```python
from build123d import *

# Parameters (mm, degrees)
F0_W     = 117.5
F0_H     = 117.5
F1_DEPTH = 150
F2_R     = 8.3617608376
F3_DEPTH = 50.8
F4_T     = -2.54


with BuildPart() as f1:
    # F0 (on Top) → F1 (new body)
    with BuildSketch(Plane.XY):
        with Locations((2.2854433954, -9.9431091547)):
            Rectangle(F0_W, F0_H)
    extrude(amount=F1_DEPTH)

    # F2 (on face) → F3 (join)
    with BuildSketch(Plane.XY.offset(150)):
        with Locations((0, 10.8060371131)):
            Circle(F2_R)
    extrude(amount=F3_DEPTH)

    # F4
    f4_openings = [f1.faces().sort_by_distance(p)[0] for p in [
        (0, 10.806037, 200.8),
    ]]
    offset(amount=F4_T, openings=f4_openings, kind=Kind.INTERSECTION)


solid = f1.part
```
Design review of the part built by this model. Coordinates are the model's own, in mm. A direction names the side the tool comes from. Give positions to 0.01 mm unless a question says otherwise; leave off trailing zeros. Order: outer loops, then holes, each group sorted by start corner. A loop starts at its lowest first (then second) coordinate and runs counter-clockwise, first axis right, second up. Notation, with made-up numbers: (82.5, 18) - (99.5, 18) arc R12 ccw to (99.5, 32) - close; hole circle Ø9 at (40.25, -35). An arc over 180 degrees is marked (long way). Use a Markdown table: item, result. Add a question column.
(1) Add section B-B on z = 76. Give the boundary of the cut face in (x, y).
(2) Mouldability with a two-part tool opening along X and no side actions: class faces 1 (the face through (-1.813, 2.643, 175.044)), 2 (the face through (1, 48.807, 74)), 3 (the face through (1, -9, 2.54)) as +X half, -X half, draft (parallel to the pull), parting line (faces both ways), or undercut.
(3) Add section C-C on y = 13. Give the boundary of the cut face in (x, z), then the cut area to 3 significant figures.
(4) Add section D-D on x = 0. Give the boundary of the cut face in (y, z).
(5) Wall thickness on probe 1 along X at (y, z) = (-19.5, 105.5); probe 2 along X at (y, z) = (11.5, 162); probe 3 along Z at (x, y) = (-46, 14): over which ranges is each line inside the solid? List them lowest first. Write a range as [from, to].
(6) Machinability: for faces 4 (the face through (-1.262, 5.123, 173.757)), 5 (the face through (58.495, -11, 74)), 6 (the face through (-56.465, -11, 74)), which of the approach directions +Z, -Z, +X, -X, +Y, -Y give a long, thin tool a straight path to every point of the face, cutting with its end or side? Answer none if there is none.
(7) Clearance check with flat-ended pins moving along their axes: P1, Ø1, axis at x = -37, y = 31.5, coming from the +Z side; P2, Ø6, axis at x = 27.5, y = 33, coming from the -Z side. State where each tip first meets the part, or that it passes through.
(8) Add section A-A on x = -44.5. Give the boundary of the cut face in (y, z), then the cut area to 3 significant figures.
Report:
| question | item | result |
|---|---|---|
| 1 | outline | (-56.46, -68.69) - (61.04, -68.69) - (61.04, 48.81) - (-56.46, 48.81) - close; hole (-53.92, -66.15) - (58.5, -66.15) - (58.5, 46.27) - (-53.92, 46.27) - close |
| 2 | face 1 | parting line |
| 2 | face 2 | draft |
| 2 | face 3 | undercut |
| 3 | outline | (-56.46, 0) - (61.04, 0) - (61.04, 150) - (8.07, 150) - (8.07, 200.8) - (5.39, 200.8) - (5.39, 147.46) - (58.5, 147.46) - (58.5, 2.54) - (-53.92, 2.54) - (-53.92, 147.46) - (-5.39, 147.46) - (-5.39, 200.8) - (-8.07, 200.8) - (-8.07, 150) - (-56.46, 150) - close |
| 3 | area | 1,580 mm² |
| 4 | outline | (-68.69, 0) - (48.81, 0) - (48.81, 150) - (19.17, 150) - (19.17, 200.8) - (16.63, 200.8) - (16.63, 147.46) - (46.27, 147.46) - (46.27, 2.54) - (-66.15, 2.54) - (-66.15, 147.46) - (4.98, 147.46) - (4.98, 200.8) - (2.44, 200.8) - (2.44, 150) - (-68.69, 150) - close |
| 5 | probe 1 | x = [-56.46, -53.92], [58.5, 61.04] |
| 5 | probe 2 | x = [-8.33, -5.78], [5.78, 8.33] |
| 5 | probe 3 | z = [0, 2.54], [147.46, 150] |
| 6 | face 4 | +Z |
| 6 | face 5 | none |
| 6 | face 6 | +Z, -Z, -X, +Y, -Y |
| 7 | P1 | stops at z = 150 |
| 7 | P2 | stops at z = 0 |
| 8 | outline | (-68.69, 0) - (48.81, 0) - (48.81, 150) - (-68.69, 150) - close; hole (-66.15, 2.54) - (46.27, 2.54) - (46.27, 147.46) - (-66.15, 147.46) - close |
| 8 | area | 1,330 mm² |
